Autodesk Fusion 360 part; units mm, degrees
sketch "Sketch1" plane through (0, 0, 0) normal (0, 1, 0) x (1, 0, 0)
  line L0 (0, 0) -> (60, 0)
  line L1 (60, 0) -> (60, -60)
  line L2 (60, -60) -> (0, -60)
  line L3 (0, -60) -> (0, 0)
  dimension "d1" = 60
  dimension "d2" = 60
extrude "Extrude1" add sketch "Sketch1" along normal blind 50
sketch "Sketch2" plane through (0, 50, 0) normal (0, 1, 0) x (-1, 0, 0)
  line L0 (0, 60) -> (-60, 60)
  line L1 (-60, 60) -> (-60, 0)
  line L2 (-60, 0) -> (0, 0)
  line L3 (0, 0) -> (0, 60)
  line L4 (-10, 10) -> (-50, 10)
  line L5 (-50, 10) -> (-50, 50)
  line L6 (-50, 50) -> (-10, 50)
  line L7 (-10, 50) -> (-10, 10)
  dimension "d5" = 10
  dimension "d6" = 10
  dimension "d7" = 10
  dimension "d8" = 10
extrude "Extrude2" cut 1 faces at (20, 0, 20) along direction (0, 1, 0) blind 20
extrude "Extrude3" cut sketch "Sketch2" against normal blind 10 contours L4 L5 L6 L7
fillet "Fillet1" radius 5 4 edges at (10, 45, 10) (10, 45, 50) (50, 45, 50) (50, 45, 10)
For this review, take the finished solid that the model builds, in its own axes (mm). A direction names the side the tool comes from. Round coordinates to 2 decimals unless told otherwise and drop trailing zeros. Write each loop counter-clockwise with the first axis right and the second up, starting at its lowest first coordinate (ties: lowest second). Pieces come first, ordered by that corner, then holes. Notation, with made-up numbers: (-35.5, 21.25) -> (-16.5, 21.25) arc R12 ccw to (-16.5, 33.25) -> close; hole circle Ø7 at (50, 81.25). An arc over 180 degrees is marked (long way). One line per question, with ' | ' between items. Start each with the question number.
1) Add section C-C (x = 48). Write out the cut boundary in (y, z), and give its area (3 significant figures).
2) Add section B-B (z = 38.5). Write out the cut boundary in (x, y), and give its area (3 significant figures).
3) Mouldability with a two-part tool opening along Z and no side actions: class faces 1 (the cylindrical face through (12, 45, 49)), 2 (the flat face through (30, 35, 60)), 3 (the flat face through (0, 35, 30)) as +Z half, -Z half, draft (parallel to the pull), parting line (faces both ways), or undercut.
4) For pin 1 Ø2 at (x, z) = (29, 21) entering from +Y, flat-tipped, find the tip position at first contact; note if it passes through.
5) Add section A-A (y = 41.25). Write out the cut boundary in (x, z).
6) Machinability: for faces 4 (the cylindrical face through (11, 45, 12)), 5 (the flat face through (30, 20, 30)), which of the approach directions +Z, -Z, +X, -X, +Y, -Y give a long, thin tool a straight path to every point of the face, cutting with its end or side? Answer none if there is none.
7) Wall thickness on line 1 along X through (y, z) = (45.75, 38); line 2 along Y through (x, z) = (38, 19): over which ranges is each line inside the solid? List them lowest first.
Reported:
1) outline: (20, 0) -> (50, 0) -> (50, 11) -> (40, 11) -> (40, 49) -> (50, 49) -> (50, 60) -> (20, 60) -> close | area: 1,420 mm²
2) outline: (0, 20) -> (60, 20) -> (60, 50) -> (50, 50) -> (50, 40) -> (10, 40) -> (10, 50) -> (0, 50) -> close | area: 1,400 mm²
3) face 1: undercut | face 2: +Z half | face 3: draft
4) pin 1: stops at y = 40
5) outline: (0, 0) -> (60, 0) -> (60, 60) -> (0, 60) -> close; hole (10, 15) arc R5 ccw to (15, 10) -> (45, 10) arc R5 ccw to (50, 15) -> (50, 45) arc R5 ccw to (45, 50) -> (15, 50) arc R5 ccw to (10, 45) -> close
6) face 4: +Y | face 5: +Z, -Z, +X, -X, -Y
7) line 1: x = 0 to 10, 50 to 60 | line 2: y = 20 to 40
